Autodesk Inventor part; units mm, degrees
ref_plane "IDS_WORKPLANE{1}" through (0, 14.2875, 0) normal (0, 1, 0) x (-1, 0, 0)
ref_plane "IDS_WORKPLANE{2}" through (6.35, 0, 0) normal (-1, 0, 0) x (0, 0, 1)
ref_plane "YZ Plane" through (0, 0, 0) normal (1, 0, 0) x (0, 1, 0)
sketch "Boceto1" plane through (0, 0, 0) normal (0, 0, 1) x (1, 0, 0)
  line L0 (0, 14.2875) -> (12.7, 14.2875)
  line L1 (-1.9497, 0) -> (21.5466, 0)
  line L2 (0, 14.2875) -> (0, 7.9375)
  line L3 (0, 7.9375) -> (12.7, 7.9375)
  line L4 (12.7, 7.9375) -> (12.7, 14.2875)
  line L5 (-6.6489, 0) -> (26.2458, 0)
  line L6 (0, 54) -> (0, -9)
  dimension "d0" = 28.575
  dimension "d1" = 15.875
  dimension "d2" = 12.7
revolve "Cuerpo" add sketch "Boceto1" angle 360 about axis through (-1.9497, 0, 0) along (1, 0, 0)
ref_plane "IDS_WORKPLANE{1}" through (0, 14.2875, 0) normal (0, 1, 0) x (-1, 0, 0)
sketch "Boceto2" plane through (0, 14.2875, 0) normal (0, 1, 0) x (-1, 0, 0)
  line L0 (0, 14.2875) -> (0, -14.2875)
  line L1 (-12.156, 0) -> (2.026, 0)
  point P0 (-6.35, 0)
  dimension "d7" = 6.35
hole "Agujero1" at (6.35, 14.2875, 0) direction (0, -1, 0) diameter 7.9375 depth 14.2875 tip angle 118
ref_plane "IDS_WORKPLANE{2}" through (6.35, 0, 0) normal (-1, 0, 0) x (0, 0, 1)
sketch "Boceto3" plane through (6.35, 0, 0) normal (-1, 0, 0) x (0, 0, 1)
  line L0 (0, 14.2875) -> (3.1293, 14.2875)
  line L1 (3.1293, 14.2875) -> (3.9688, 14.1091)
  line L2 (3.9688, 14.1091) -> (3.9688, 8.8946)
  line L3 (0, 56.8575) -> (0, -26.145)
  circle A0 centre (0, 0) radius 14.2875
  line L4 (0, 14.2875) -> (0, 7.9375)
  line L5 (3.9688, 8.8946) -> (0.3969, 7.9375)
  line L6 (0.3969, 7.9375) -> (0, 7.9375)
  dimension "d18" = 6.2586
  dimension "d19" = 7.9375
  dimension "d20" = 0.7937
  dimension "d21" = 6.35
  dimension "d30" = 15
  dimension "d31" = 12
revolve "Tornillo de cabeza perdida1" add sketch "Boceto3" angle 360 about axis through (6.35, 14.2875, 0) along (0, -1, 0) picked at (1.9014, 10.3523) contours A0 L2 L5 L6 L3 | L0 L1 L2 A0
sketch "Boceto4" plane through (0, 14.2875, 0) normal (0, 1, 0) x (-1, 0, 0)
  line L0 (-6.35, 1.5875) -> (-4.9752, 0.7937)
  line L1 (-4.9752, 0.7937) -> (-4.9752, -0.7938)
  line L2 (-4.9752, -0.7938) -> (-6.35, -1.5875)
  line L3 (-6.35, -1.5875) -> (-7.7248, -0.7937)
  line L4 (-7.7248, -0.7937) -> (-7.7248, 0.7938)
  line L5 (-7.7248, 0.7938) -> (-6.35, 1.5875)
  line L6 (-14.2345, 0) -> (2.3724, 0)
  line L7 (0, 7.9375) -> (0, -7.9375)
  point P0 (-6.35, 0)
  dimension "d22" = 3.175
  dimension "d23" = 6.35
extrude "Ranura1" cut sketch "Boceto4" against normal blind 1.9844
chamfer "Chaflán1" distance 1.27 angle 15 1 edges at (12.7, -14.2875, 0) measured on face at (4.2333, 9.0361, 11.0672)
chamfer "Chaflán2" distance 0.2381 distance2 1.27 1 edges at (12.7, -7.9375, 0) measured on face at (12.7, 11.8089, -1.1126)
fillet "Empalme1" radius 0.635 1 edges at (0, -14.2875, 0)
equation "\"d18\" = GD1"
equation "\"d19\" = NND"
equation "\"d20\" = 0.1 * NND"
equation "\"d21\" = -0.5 * WND + 0.5 * SD2"
equation "\"d30\" = FAWI"
equation "\"d31\" = 0.8 * FAWI"
equation "\"d22\" = 0.4 * NND"
equation "\"d24\" = 0.25 * NND"
equation "\"d8\" = NND"
equation "\"d13\" = 0.5 * SD2"
equation "\"d4\" = PHH"
equation "\"d5\" = FAWI"
equation "\"d59\" = PHH"
equation "\"d26\" = -0.5 * WND + 0.5 * NND1"
equation "\"d27\" = PHH"
equation "\"d29\" = RR"
equation "\"d0\" = SD2"
equation "\"d1\" = WND"
equation "\"d2\" = SD"
equation "\"WND\" = 15.875"
equation "\"SD2\" = 28.575"
equation "\"SD\" = 12.7"
equation "\"NND\" = 7.9375"
equation "\"FAWI\" = 15deg"
equation "\"PHH\" = 1.27"
equation "\"d6\" = 0.5 * SD2"
equation "\"GD1\" = 6.25856"
equation "\"d17\" = -0.5 * SD"
equation "\"RR\" = 0.635"
equation "\"NND1\" = 16.35125"
properties part number "Unbrako. Hallowell Steel Collars. Inch Series - 0.625 x 1 1/8 x 1/2" material "Acero, suave"
Part model, mm, in its own coordinate system. A direction names the side the tool comes from. Give positions to 0.01 mm unless a question says otherwise; leave off trailing zeros. Loops run counter-clockwise (first coordinate to the right, second up) from the corner with the lowest first, then second, coordinate; pieces in that order, holes last. Notation, with made-up numbers: M -35,-32.75 L 10,-32.75 A17 cw 10,-10.75 Z; hole C 64,-14 d3. An arc over 180 degrees is marked long. Put each result on its own line as item: value. Start each with the question number.
1) 3-axis set-ups, long thin cutter, end or side, ignore diameter. For faces 5 (the cylindrical face through (6.296, 13.957, -3.968)), 6 (the cylindrical face through (3.668, 8.095, -2.925)), 7 (the flat face through (4.975, 13, 0)): which of +Z, -Z, +X, -X, +Y, -Y reach the whole face in a straight line?
2) Saw through at A-A (y = 0). List the corners of the cut face in (x, z) (1 decimal), then the cut area to 3 significant figures.
3) Pull direction X, two halves, no side cores. Call faces 1 (the flat face through (6, 12.303, 0)), 2 (the flat face through (5.61, 14.288, 1.35)), 3 (the cylindrical face through (6.404, 13.957, 3.968)), 4 (the conical face through (5.8, 8, 0.3)): +X half, -X half, draft (parallel to the pull), parting line (faces both ways), or undercut.
4) Flat gauge pins, fed straight in: pin 1 (4 mm diameter, centred on x = 10.5, y = -7.5, fed in from -Z); pin 2 (4 mm diameter, centred on x = 11.5, y = 3, fed in from +Z); pin 3 (3 mm diameter, centred on x = 4.5, z = -11.5, fed in from -Y); pin 4 (2 mm diameter, centred on y = -3, z = -5.5, fed in from +X). Where does each tip first touch, or does it go through?
5) Probe probe 1 along Z at (x, y) = (5.75, 0); probe 2 along Y at (x, z) = (6, -0.25); probe 3 along Y at (x, z) = (11.5, -0.5). List the from-to ranges inside material, lowest first.
Numbers:
1. face 5: -Z, +Y
1. face 6: none
1. face 7: +Y
2. outline: M 0,-13.7 A0.6 ccw 0.6,-14.3 L 11.4,-14.3 L 12.7,-13.9 L 12.7,-8.2 L 11.4,-7.9 L 0,-7.9 Z; M 0,7.9 L 11.4,7.9 L 12.7,8.2 L 12.7,13.9 L 11.4,14.3 L 0.6,14.3 A0.6 ccw 0,13.7 Z
2. area: 160 mm^2
3. face 1: undercut
3. face 2: draft
3. face 3: parting line
3. face 4: undercut
4. pin 1: z = -13.19
4. pin 2: z = 14.25
4. pin 3: y = -10.2
4. pin 4: through
5. probe 1: -14.29 to -7.94, 7.94 to 14.29
5. probe 2: -14.29 to -7.93, 7.95 to 12.3
5. probe 3: -14.26 to -7.93, 7.93 to 14.26
